```python
from build123d import *

# Parameters (mm, degrees)
BOX008_W          = 8
BOX008_H          = 55
BOX008_DEPTH      = 37
CYLINDER022_R     = 4.1
CYLINDER022_DEPTH = 12
CYLINDER010_R     = 4.1
CYLINDER010_DEPTH = 12
CYLINDER006_R     = 4.5
CYLINDER006_DEPTH = 5
CYLINDER005_R     = 2.5
CYLINDER005_DEPTH = 5
CYLINDER012_R     = 4.5
CYLINDER012_DEPTH = 5
CYLINDER011_R     = 2.5
CYLINDER011_DEPTH = 5
BOX_W             = 10
BOX_H             = 12
BOX_DEPTH         = 83


with BuildPart() as obj1:
    # Box008 → Box008 (new body)
    with BuildSketch(Plane(origin=(34, -21, 0), x_dir=(1, 0, 0), z_dir=(0, 0, 1))):
        with Locations((4, 27.5)):
            Rectangle(BOX008_W, BOX008_H)
    extrude(amount=BOX008_DEPTH)


with BuildPart() as obj2:
    # Cylinder022 → Cylinder022 (new body)
    with BuildSketch(Plane(origin=(32, 12, 73), x_dir=(1, 0, 0), z_dir=(0, -1, 0))):
        Circle(CYLINDER022_R)
    extrude(amount=CYLINDER022_DEPTH)


with BuildPart() as obj3:
    # Cylinder010 → Cylinder010 (new body)
    with BuildSketch(Plane(origin=(32, 12, 55), x_dir=(1, 0, 0), z_dir=(0, -1, 0))):
        Circle(CYLINDER010_R)
    extrude(amount=CYLINDER010_DEPTH)


with BuildPart() as cylinder006:
    # Cylinder006 → Cylinder006 (new body)
    with BuildSketch(Plane(origin=(37, 5, 55), x_dir=(0, 0, -1), z_dir=(1, 0, 0))):
        Circle(CYLINDER006_R)
    extrude(amount=CYLINDER006_DEPTH)


with BuildPart() as obj4:
    # Cylinder005 → Cylinder005 (new body)
    with BuildSketch(Plane(origin=(32, 5, 55), x_dir=(0, 0, -1), z_dir=(1, 0, 0))):
        Circle(CYLINDER005_R)
    extrude(amount=CYLINDER005_DEPTH)

    # Fusion003: union Cylinder006
    add(cylinder006.part)


with BuildPart() as obj4_1:
    # Fusion003 placement: moved
    add(obj4.part.moved(Location((0, 1, 9))))


with BuildPart() as cylinder012:
    # Cylinder012 → Cylinder012 (new body)
    with BuildSketch(Plane(origin=(37, 5, 55), x_dir=(0, 0, -1), z_dir=(1, 0, 0))):
        Circle(CYLINDER012_R)
    extrude(amount=CYLINDER012_DEPTH)


with BuildPart() as screwholes:
    # Cylinder011 → Cylinder011 (new body)
    with BuildSketch(Plane(origin=(32, 5, 55), x_dir=(0, 0, -1), z_dir=(1, 0, 0))):
        Circle(CYLINDER011_R)
    extrude(amount=CYLINDER011_DEPTH)

    # Fusion004: union Cylinder012
    add(cylinder012.part)


with BuildPart() as screwholes_1:
    # Fusion004 placement: moved
    add(screwholes.part.moved(Location((0, 1, -11))))

    # Fusion005: union obj4
    add(obj4_1.part)


with BuildPart() as obj5:
    # Box → Box (new body)
    with BuildSketch(Plane(origin=(32, 0, 0), x_dir=(1, 0, 0), z_dir=(0, 0, 1))):
        with Locations((5, 6)):
            Rectangle(BOX_W, BOX_H)
    extrude(amount=BOX_DEPTH)

    # Cut: cut ScrewHoles
    add(screwholes_1.part, mode=Mode.SUBTRACT)

    # Cut007: cut obj3
    add(obj3.part, mode=Mode.SUBTRACT)

    # Cut008: cut obj2
    add(obj2.part, mode=Mode.SUBTRACT)

    # Fusion011: union obj1
    add(obj1.part)


solid = obj5.part
```
Could you check a few things on this model? Use its own coordinates, in mm. A direction names the side the tool comes from. Round coordinates to 2 decimals unless told otherwise and drop trailing zeros. Loops run counter-clockwise (first coordinate to the right, second up) from the corner with the lowest first, then second, coordinate; pieces in that order, holes last.
Q1. Thinking about a two-plate mould opening in Z: for faces 1 (the flat face through (37, 6, 83)), 2 (the cylindrical face through (34.465, 6.751, 41.615)), 3 (the cylindrical face through (34.465, 6.751, 61.615)), 4 (the flat face through (32, 6, 25)), which applies, pulls with the +Z half, pulls with the -Z half, needs draft (parallel to the pull), parting line crosses it, or undercut?
Q2. I want a section at A-A (y = 7.5). Write out the boundary of the cut face in (x, z).
Q3. I want a section at C-C (x = 33). Write out the boundary of the cut face in (y, z), and give its area (3 significant figures).
Q4. For P1, Ø7, axis at y = 6, z = 44, coming from the +X side; P2, Ø3, axis at y = 6, z = 64, coming from the -X side; P3, Ø17.5, axis at y = 25.5, z = 20.5, coming from the -X side; P4, Ø5, axis at x = 37, z = 40.5, coming from the -Y side, each with a flat end and sliding along its axis, tell me the tip position at first contact or that it passes through.
Q5. I want a section at D-D (z = 30.5). Write out the boundary of the cut face in (x, y).
Q6. I want a section at B-B (z = 44). Write out the boundary of the cut face in (x, y).
Q7. On a 3-axis mill with a long thin cutter (end or side, diameter ignored), from which of +Z, -Z, +X, -X, +Y, -Y can I reach the whole of each face in a straight line? I mean faces 5 (the flat face through (38, -10, 37)), 6 (the cylindrical face through (39.465, 7.352, 39.708)), 7 (the flat face through (38, 23, 37)). Say none if no direction works.
Q8. Please list where these lines run through material, in increasing order: L1, parallel to Y at x = 38.3, z = 64; L2, parallel to Y at x = 34.5, z = 64; L3, parallel to Z at x = 35.5, y = -10.
Answer below:
1. face 1: pulls with the +Z half
1. face 2: undercut
1. face 3: undercut
1. face 4: needs draft
2. outline: (32, 0) - (42, 0) - (42, 39.76) - (37, 39.76) - (37, 42) - (32, 42) - close; (32, 46) - (37, 46) - (37, 48.24) - (42, 48.24) - (42, 59.76) - (37, 59.76) - (37, 62) - (32, 62) - (32, 59.1) arc R4.1 cw to (32, 50.9) - close; (32, 66) - (37, 66) - (37, 68.24) - (42, 68.24) - (42, 83) - (32, 83) - (32, 77.1) arc R4.1 cw to (32, 68.9) - close
3. outline: (0, 0) - (12, 0) - (12, 51.02) - (0, 51.02) - close; (0, 58.98) - (12, 58.98) - (12, 69.02) - (0, 69.02) - close; (0, 76.98) - (12, 76.98) - (12, 83) - (0, 83) - close; hole circle Ø5 at (6, 44); hole circle Ø5 at (6, 64)
3. area: 766 mm2
4. P1: stops at x = 37
4. P2: passes through
4. P3: stops at x = 34
4. P4: stops at y = 0
5. outline: (32, 0) - (34, 0) - (34, -21) - (42, -21) - (42, 34) - (34, 34) - (34, 12) - (32, 12) - close
6. outline: (32, 0) - (42, 0) - (42, 1.5) - (37, 1.5) - (37, 3.5) - (32, 3.5) - close; (32, 8.5) - (37, 8.5) - (37, 10.5) - (42, 10.5) - (42, 12) - (32, 12) - close
7. face 5: +Z, +X, -X, -Y
7. face 6: +X
7. face 7: +Z, +X, -X, +Y
8. L1: y = 0 to 1.5, 10.5 to 12
8. L2: y = 0 to 3.5, 8.5 to 12
8. L3: z = 0 to 37
